```python
from build123d import *

# Parameters (mm, degrees)
SKETCH1_R           = 22.225
SKETCH1_R_2         = 16.129
BOSS_EXTRUDE1_DEPTH = 8.2
CIRPATTERN1_COUNT   = 6


with BuildPart() as part:
    # Sketch1 → Boss-Extrude1 (new body)
    with BuildSketch(Plane.XY):
        Circle(SKETCH1_R)
        Circle(SKETCH1_R_2, mode=Mode.SUBTRACT)
    extrude(amount=BOSS_EXTRUDE1_DEPTH)

    # Sketch2 → 3/32 (0.09375) Diameter Hole1 (revolve, cut)
    with BuildSketch(Plane(origin=(0, 19.05, 8.2), x_dir=(0, -1, 0), z_dir=(1, 0, 0))):
        Polygon((0, 0), (0, 26.115399675), (1.190625, 25.4), (1.190625, 0), align=None)
    f_3_32_0_09375_diameter_hole1 = revolve(axis=Axis((0, 19.05, 14.55), (0, 0, -1)), mode=Mode.SUBTRACT)

    # CirPattern1: 3/32 (0.09375) Diameter Hole1 ×6 about axis
    cirpattern1_axis = Axis((0, 0, 0), (0, 0, 1))
    for i in range(1, CIRPATTERN1_COUNT):
        add(f_3_32_0_09375_diameter_hole1.rotate(cirpattern1_axis, i * 360 / CIRPATTERN1_COUNT), mode=Mode.SUBTRACT)


solid = part.part
```
Check sheet for the modelled part. Datum: model origin and axes. Units: mm. Coordinates: 2 decimals unless noted, no trailing zeros. Write each loop counter-clockwise with the first axis right and the second up, starting at its lowest first coordinate (ties: lowest second). Pieces come first, ordered by that corner, then holes. Notation, with made-up numbers: M 77.25,84.25 L 113.25,84.25 A22 cw 113.25,122.25 Z; hole C 88.25,-13 d1. An arc over 180 degrees is marked long. Write item = value, one per line. Start each with the question number.
1. Go/stop test with flat-tipped pins: pin 1 (2 mm diameter, centred on x = -1.5, z = 1, fed in from -Y); pin 2 (4 mm diameter, centred on x = 7.5, z = 6.5, fed in from -Y); pin 3 (1.4 mm diameter, centred on x = 0, y = 19.05, fed in from +Z); pin 4 (1 mm diameter, centred on y = 2, z = 5.5, fed in from -X). Record where each tip stops, or that it passes through.
2. Mould release check, pull along X, two halves, no side actions. Record for faces 1 (the cylindrical face through (-15.773, -8.58, 4.157)), 2 (the cylindrical face through (21.199, 6.676, 4.043)), 3 (the flat face through (15, 7, 0)): pulls with the +X half, pulls with the -X half, needs draft (parallel to the pull), parting line crosses it, or undercut.
3. Sectioned sample at C-C (x = 0). Record the cut outline in (y, z) (3 decimals), then the cut area to 3 significant figures.
4. Sectioned sample at B-B (x = -8.5). Record the cut outline in (y, z).
5. Sectioned sample at D-D (z = 5.25). Record the cut outline in (x, y) (3 decimals).
6. Sectioned sample at A-A (y = 0). Record the cut outline in (x, z) (3 decimals).
7. Thickness scan on probe 1 along Y at (x, z) = (0, 6.5) (3 decimals); probe 2 along Y at (x, z) = (9, 4.5); probe 3 along Y at (x, z) = (3.5, 6). Record the ranges inside material, lowest first.
The answers:
q1.pin_1 = -22.22
q1.pin_2 = -21.53
q1.pin_3 = through
q1.pin_4 = -22.17
q2.face_1 = undercut
q2.face_2 = parting line crosses it
q2.face_3 = needs draft
q3.outline = M -22.225,0 L -20.241,0 L -20.241,8.2 L -22.225,8.2 Z; M -17.859,0 L -16.129,0 L -16.129,8.2 L -17.859,8.2 Z; M 16.129,0 L 17.859,0 L 17.859,8.2 L 16.129,8.2 Z; M 20.241,0 L 22.225,0 L 22.225,8.2 L 20.241,8.2 Z
q3.area = 60.9 mm²
q4.outline = M -20.54,0 L -13.71,0 L -13.71,8.2 L -20.54,8.2 Z; M 13.71,0 L 20.54,0 L 20.54,8.2 L 13.71,8.2 Z
q5.outline = C 0,0 d44.45; hole C -16.498,-9.525 d2.381; hole C -16.498,9.525 d2.381; hole C 0,0 d32.258; hole C 0,-19.05 d2.381; hole C 0,19.05 d2.381; hole C 16.498,-9.525 d2.381; hole C 16.498,9.525 d2.381
q6.outline = M -22.225,0 L -16.129,0 L -16.129,8.2 L -22.225,8.2 Z; M 16.129,0 L 22.225,0 L 22.225,8.2 L 16.129,8.2 Z
q7.probe_1 = -22.225 to -20.241, -17.859 to -16.129, 16.129 to 17.859, 20.241 to 22.225
q7.probe_2 = -20.32 to -13.38, 13.38 to 20.32
q7.probe_3 = -21.95 to -15.74, 15.74 to 21.95
